Here's how the part is built. I have some questions about the finished solid (model axes, mm). Face numbers are marked on the shaded views. A direction names the side the tool comes from. Coordinates: 2 decimals unless noted, no trailing zeros. Write each loop counter-clockwise with the first axis right and the second up, starting at its lowest first coordinate (ties: lowest second). Pieces come first, ordered by that corner, then holes.
```python
from build123d import *

# Parameters (mm, degrees)
SKETCH1_R           = 8.985
BOSS_EXTRUDE1_DEPTH = 1.12
SKETCH2_R           = 7.985
BOSS_EXTRUDE2_DEPTH = 3.88
SKETCH3_R           = 2.42
CUT_EXTRUDE1_DEPTH  = 6
SKETCH4_R           = 6.5
SKETCH4_R_2         = 4.5
CUT_EXTRUDE2_DEPTH  = 0.08
SKETCH5_R           = 6.5
SKETCH5_R_2         = 4.5
CUT_EXTRUDE3_DEPTH  = 0.08
FILLET1_R           = 0.31


with BuildPart() as part:
    # Sketch1 → Boss-Extrude1 (new body)
    with BuildSketch(Plane(origin=(0, 0, 0), x_dir=(1, 0, 0), z_dir=(0, 1, 0))):
        Circle(SKETCH1_R)
    extrude(amount=BOSS_EXTRUDE1_DEPTH)

    # Sketch2 → Boss-Extrude2 (add)
    with BuildSketch(Plane(origin=(0, 1.12, 0), x_dir=(1, 0, 0), z_dir=(0, 1, 0))):
        Circle(SKETCH2_R)
    extrude(amount=BOSS_EXTRUDE2_DEPTH)

    # Sketch3 → Cut-Extrude1 (cut, through all)
    with BuildSketch(Plane(origin=(0, 5, 0), x_dir=(1, 0, 0), z_dir=(0, 1, 0))):
        Circle(SKETCH3_R)
    extrude(amount=-CUT_EXTRUDE1_DEPTH, mode=Mode.SUBTRACT)

    # Sketch4 → Cut-Extrude2 (cut)
    with BuildSketch(Plane.XZ):
        Circle(SKETCH4_R)
        Circle(SKETCH4_R_2, mode=Mode.SUBTRACT)
    extrude(amount=-CUT_EXTRUDE2_DEPTH, mode=Mode.SUBTRACT)

    # Sketch5 → Cut-Extrude3 (cut)
    with BuildSketch(Plane(origin=(0, 5, 0), x_dir=(1, 0, 0), z_dir=(0, 1, 0))):
        Circle(SKETCH5_R)
        Circle(SKETCH5_R_2, mode=Mode.SUBTRACT)
    extrude(amount=-CUT_EXTRUDE3_DEPTH, mode=Mode.SUBTRACT)

    # Fillet1
    fillet1_edges = [part.edges().sort_by_distance(p)[0] for p in [
        (-2.42, 0, 0),
        (-2.42, 5, 0),
        (-8.985, 0, 0),
        (-7.985, 5, 0),
    ]]
    fillet(fillet1_edges, radius=FILLET1_R)


solid = part.part
```
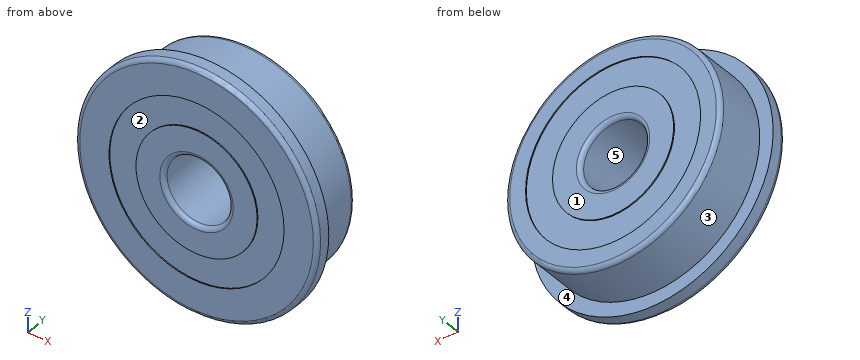
1) On a 3-axis mill with a long thin cutter (end or side, diameter ignored), from which of +Z, -Z, +X, -X, +Y, -Y can I reach the whole of each face in a straight line? I mean the marked faces 4 and 5. Say none if no direction works.
Values follow:
face 4: +Y
face 5: +Y, -Y
2) Imagine slicing it at A-A on y = 1.4. Please give me the cut outline in (x, z) (3 decimals), then the cut area to 3 significant figures.
Values follow:
outline: circle Ø15.97 at (0, 0); hole circle Ø4.84 at (0, 0)
area: 182 mm2
3) We'd pull the mould along X, two halves only. Please class the marked faces 1, 2 and 3: pulls with the +X half, pulls with the -X half, needs draft (parallel to the pull), parting line crosses it, or undercut.
Values follow:
face 1: needs draft
face 2: undercut
face 3: parting line crosses it
4) Will these pins go through, and if not, where does the flat tip stop? pin 1 (3 mm diameter, centred on x = -2, y = 2.5, fed in from +Z); pin 2 (2 mm diameter, centred on x = -3.5, y = 3.5, fed in from -Z); pin 3 (1.5 mm diameter, centred on x = -1, z = 1, fed in from -Y); pin 4 (3 mm diameter, centred on x = -2, y = 1.5, fed in from -Z).
Values follow:
pin 1: stops at z = 8.87
pin 2: stops at z = -7.58
pin 3: passes through
pin 4: stops at z = -8.97
5) I need wall thicknesses on probe 1 along X at (y, z) = (2.75, 0) (3 decimals); probe 2 along Y at (x, z) = (-8, -2). Which ranges of each line are inside material? Lowest first, please.
Values follow:
probe 1: x = -7.985 to -2.42, 2.42 to 7.985
probe 2: y = 0 to 1.12
